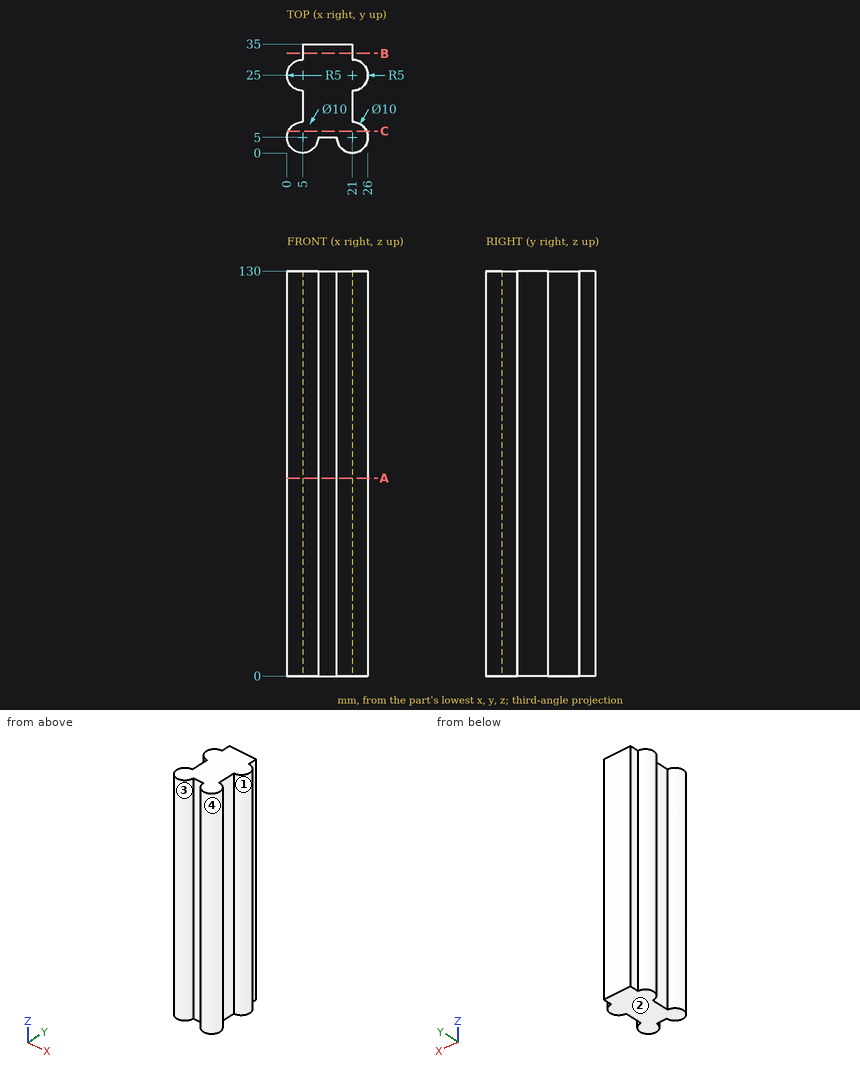
Answer from the drawing. Dimensions are ordinates in mm from the lowest x, y and z of the part. Round coordinates to 2 decimals unless told otherwise and drop trailing zeros. Write each loop counter-clockwise with the first axis right and the second up, starting at its lowest first coordinate (ties: lowest second). Pieces come first, ordered by that corner, then holes.
1. The part is cut by section A-A, the plane z = 63.5. Determine the outline of the cut face in (x, y).
2. The part is cut by section B-B, the plane y = 32. Determine the outline of the cut face in (x, z), then the cut area to 3 significant figures.
3. Given pin 1 Ø12 at (y, z) = (9, 34) entering from +X; pin 2 Ø1.5 at (y, z) = (32, 91) entering from -X; pin 3 Ø5.5 at (y, z) = (32, 63.5) entering from +X; pin 4 Ø5 at (y, z) = (14.5, 94) entering from +X, each flat-ended and moving along its own axis, determine where each tip first touches the part or whether it passes through.
4. Straight lines are drawn through the part: L1, parallel to X at y = 4, z = 111; L2, parallel to X at y = 16.5, z = 86.5; L3, parallel to Y at x = 12.5, z = 40. For each, find the intervals that lie inside material, in ascending order.
5. The part is cut by section C-C, the plane y = 7. Determine the outline of the cut face in (x, z), then the cut area to 3 significant figures.
6. Determine the mould class of the marked faces 1, 2, 3 and 4 for opening direction X: pulls with the +X half, pulls with the -X half, needs draft (parallel to the pull), parting line crosses it, or undercut.
Values:
1. outline: (5, 10) arc R5 ccw (long way) to (10, 5) - (16, 5) arc R5 ccw (long way) to (21, 10) - (21, 20) arc R5 ccw to (21, 30) - (21, 35) - (5, 35) - (5, 30) arc R5 ccw to (5, 20) - close
2. outline: (5, 0) - (21, 0) - (21, 130) - (5, 130) - close
2. area: 2,080 mm2
3. pin 1: stops at x = 26
3. pin 2: stops at x = 5
3. pin 3: stops at x = 23.63
3. pin 4: stops at x = 21
4. L1: x = 0.1 to 9.9, 16.1 to 25.9
4. L2: x = 5 to 21
4. L3: y = 5 to 35
5. outline: (0.42, 0) - (25.58, 0) - (25.58, 130) - (0.42, 130) - close
5. area: 3,270 mm2
6. face 1: pulls with the +X half
6. face 2: needs draft
6. face 3: undercut
6. face 4: undercut
